from build123d import *

# Parameters (mm, degrees)
F0_R     = 15
F1_DEPTH = 5
F2_R     = 15
F2_R_2   = 13
F3_DEPTH = 3


# Not quite as in the source:
# - a feature names something its author has since deleted; it is built from what else it names


with BuildPart() as f1:
    # F0 (on Right) → F1 (new body, symmetric)
    with BuildSketch(Plane.YZ):
        Circle(F0_R)
    extrude(amount=F1_DEPTH, both=True)

    # F2 (on Right) → F3 (cut, symmetric)
    with BuildSketch(Plane.YZ):
        Circle(F2_R)
        Circle(F2_R_2, mode=Mode.SUBTRACT)
    extrude(amount=F3_DEPTH, both=True, mode=Mode.SUBTRACT)


solid = f1.part
The model under review builds one solid part; all positions refer to its coordinate system, in mm. A direction names the side the tool comes from. Round coordinates to 2 decimals unless told otherwise and drop trailing zeros. Order: outer loops, then holes, each group sorted by start corner. A loop starts at its lowest first (then second) coordinate and runs counter-clockwise, first axis right, second up. Notation, with made-up numbers: (-9, 7) -> (23, 7) arc R30 ccw to (23, 32) -> close; hole circle Ø10 at (40.5, 24.25). An arc over 180 degrees is marked (long way). Write item = value, one per line. Start each with the question number.
Item 1: Consider section A-A on z = 0. Write out the cut boundary in (x, y), plus the area to 3 significant figures.
Item 2: Clearance check with flat-ended pins moving along their axes: pin 1 Ø2 at (x, y) = (1, 1.5) entering from -Z; pin 2 Ø5 at (x, y) = (-2, 4) entering from -Z; pin 3 Ø1.5 at (x, y) = (-2.5, 8.5) entering from +Z. State where each tip first meets the part, or that it passes through.
Item 3: For line 1 along X through (y, z) = (-12.75, -6.5); line 2 along Y through (x, z) = (0.25, 4.75); line 3 along Z through (x, y) = (-2.5, -5.5), list the stretches that pass through material, from the lowest coordinate up.
Item 4: For faces 4 (the face through (5, 0, 0)), 5 (the face through (-3, -0.1, 13.4)), list the 3-axis set-ups (+Z, -Z, +X, -X, +Y, -Y) from which the entire face can be reached by the end or side of a thin tool; tool diameter is ignored.
Item 5: Consider section C-C on x = -0.25. Write out the cut boundary in (y, z).
Item 6: Consider section D-D on x = -4. Write out the cut boundary in (y, z), plus the area to 3 significant figures.
Item 7: Mouldability with a two-part tool opening along X and no side actions: class faces 1 (the face through (-0.042, -10.316, -7.91)), 2 (the face through (4.014, -14.985, 0.66)), 3 (the face through (-5, 0, 0)) as released by +X, released by -X, zero draft, split by the parting line, or undercut.
Conclusion:
q1.outline = (-5, -15) -> (-3, -15) -> (-3, -13) -> (3, -13) -> (3, -15) -> (5, -15) -> (5, 15) -> (3, 15) -> (3, 13) -> (-3, 13) -> (-3, 15) -> (-5, 15) -> close
q1.area = 276 mm2
q2.pin_1 = -12.99
q2.pin_2 = -14.9
q2.pin_3 = 12.73
q3.line_1 = -5 to -3, 3 to 5
q3.line_2 = -12.1 to 12.1
q3.line_3 = -11.78 to 11.78
q4.face_4 = +Z, -Z, +X, +Y, -Y
q4.face_5 = none
q5.outline = circle Ø26 at (0, 0)
q6.outline = circle Ø30 at (0, 0)
q6.area = 707 mm2
q7.face_1 = undercut
q7.face_2 = zero draft
q7.face_3 = released by -X
